The listing builds one solid part. Answer for the finished solid, in the listing's coordinates (mm). Face numbers are marked on the shaded views. A direction names the side the tool comes from. Round coordinates to 2 decimals unless told otherwise and drop trailing zeros. Write each loop counter-clockwise with the first axis right and the second up, starting at its lowest first coordinate (ties: lowest second). Pieces come first, ordered by that corner, then holes. Notation, with made-up numbers: M -23.75,-6.75 L -13.75,-6.75 A22 cw -13.75,20.25 Z; hole C 28,39 d9. An arc over 180 degrees is marked long. Put each result on its own line as item: value. Start each with the question number.
```python
from build123d import *

# Parameters (mm, degrees)
CUT_EXTRUDE1_DEPTH = 1.117599032


with BuildPart() as part:
    # Sketch1 → Base-Revolve (revolve)
    with BuildSketch(Plane.XY, mode=Mode.PRIVATE) as base_revolve_sk:
        with BuildLine():
            Line((0, 0), (3.327397118, 0))
            Line((3.327397118, 0), (3.327397118, 0.38099967))
            ThreePointArc((3.327397118, 0.38099967), (2.644648832, 1.229467376), (1.752598482, 1.854198394))
            Line((1.752598482, 1.854198394), (0, 1.854198394))
            Line((0, 1.854198394), (0, 0))
        make_face()
    revolve(base_revolve_sk.sketch.rotate(Axis((0, 0, 0), (0, 1, 0)), 90), axis=Axis((0, 0, 0), (0, 1, 0)))

    # Sketch2 → Boss-Revolve1 (revolve)
    with BuildSketch(Plane.XY, mode=Mode.PRIVATE) as boss_revolve1_sk:
        Polygon((0, -6.3499945), (1.280158891, -6.3499945), (1.752598482, -5.877554909), (1.752598482, 0), (0, 0), align=None)
    revolve(boss_revolve1_sk.sketch.rotate(Axis((0, 0, 0), (0, 1, 0)), 90), axis=Axis((0, 0, 0), (0, 1, 0)))

    # Sketch3 → Cut-Extrude1 (cut)
    with BuildSketch(Plane(origin=(0, 1.854198394, 0), x_dir=(-1, 0, 0), z_dir=(0, 1, 0))):
        Polygon((0.990599142, 0.571922681), (0, 1.143845363), (-0.990599142, 0.571922681), (-0.990599142, -0.571922681), (0, -1.143845363), (0.990599142, -0.571922681), align=None)
    extrude(amount=-CUT_EXTRUDE1_DEPTH, mode=Mode.SUBTRACT)


solid = part.part
```
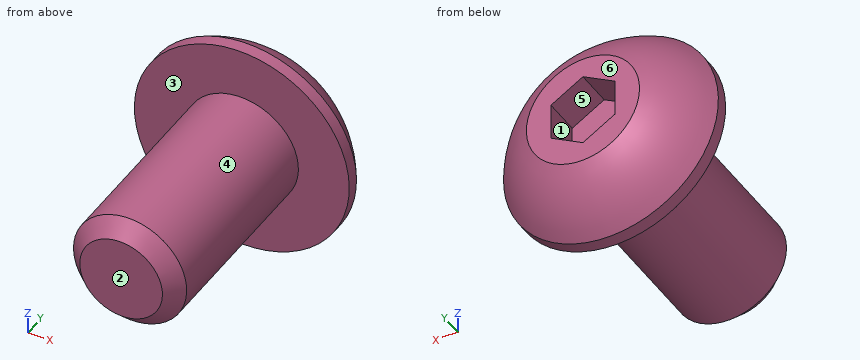
Item 1: Flat-ended cylindrical pins translate along their axes: pin 1 (2 mm diameter, centred on y = -0.5, z = -2.5, fed in from +X); pin 2 (3 mm diameter, centred on y = -4.5, z = -0.5, fed in from -X); pin 3 (0.6 mm diameter, centred on x = 0, z = 0, fed in from +Y). Find the tip coordinate at first contact, or state that the pin passes through.
Item 2: Section A-A (z = 0) is taken. Give the vertices of the cut face in (x, y), and give its area (3 significant figures).
Item 3: Section C-C (x = 2.5) is taken. Give the vertices of the cut face in (y, z).
Item 4: Consider line 1 along X through (y, z) = (1, 0); line 2 along X through (y, z) = (1, 0.75); line 3 along Y through (x, z) = (0.25, 0). Determine where each line is inside the solid, lowest interval first. Write a range as [from, to].
Item 5: Section D-D (x = -3) is taken. Give the vertices of the cut face in (y, z).
Item 6: Which of the six approach directions +Z, -Z, +X, -X, +Y, -Y give full straight-line access (tool end or side, diameter ignored) to the marked faces 1, 2 and 3?
Item 7: Section B-B (y = -1.5) is taken. Give the vertices of the cut face in (x, z).
Item 8: Determine the mould class of the marked faces 4, 5 and 6 for opening direction X: released by +X, released by -X, zero draft, split by the parting line, or undercut.
Output values:
1. pin 1: stops at x = 2.9
1. pin 2: stops at x = -1.75
1. pin 3: stops at y = 0.74
2. outline: M -3.33,0 L -1.75,0 L -1.75,-5.88 L -1.28,-6.35 L 1.28,-6.35 L 1.75,-5.88 L 1.75,0 L 3.33,0 L 3.33,0.38 A3.87 ccw 1.75,1.85 L 0.99,1.85 L 0.99,0.74 L -0.99,0.74 L -0.99,1.85 L -1.75,1.85 A3.87 ccw -3.33,0.38 Z
2. area: 30.3 mm^2
3. outline: M 0,-2.2 L 0.38,-2.2 A2.96 ccw 0.38,2.2 L 0,2.2 Z
4. line 1: x = [-2.87, -0.99], [0.99, 2.87]
4. line 2: x = [-2.77, -0.68], [0.68, 2.77]
4. line 3: y = [-6.35, 0.74]
5. outline: M 0,-1.44 L 0.38,-1.44 A2.45 ccw 0.38,1.44 L 0,1.44 Z
6. face 1: +Y
6. face 2: +Z, -Z, +X, -X, -Y
6. face 3: -Y
7. outline: C 0,0 d3.51
8. face 4: split by the parting line
8. face 5: undercut
8. face 6: zero draft
